Source: CAD feature listing. Evaluate the final solid. Frame: model axes, mm. Round coordinates to 2 decimals unless told otherwise and drop trailing zeros. Write each loop counter-clockwise with the first axis right and the second up, starting at its lowest first coordinate (ties: lowest second). Pieces come first, ordered by that corner, then holes. Notation, with made-up numbers: M -12.75,44.5 L 35.25,44.5 A22 ccw 35.25,69.5 Z; hole C 76,82 d3. An arc over 180 degrees is marked long. Use a Markdown table: item, result.
```python
from build123d import *

# Parameters (mm, degrees)
SKETCH_1_R      = 11.25
EXTRUDE_1_DEPTH = 15
SKETCH_2_R      = 5
EXTRUDE_2_DEPTH = 31
CHAMFER_1_SIZE  = 1
F_6_0MM_2_D     = 6


with BuildPart() as part:
    # 草图1 → 凸台-拉伸1 (new body)
    with BuildSketch(Plane(origin=(0, 0, 0), x_dir=(1, 0, 0), z_dir=(0, 1, 0))):
        with Locations(Location((0, 0, 0), (0, 0, 270))):
            Circle(SKETCH_1_R)
    extrude(amount=EXTRUDE_1_DEPTH)

    # 草图2 → 凸台-拉伸2 (add)
    with BuildSketch(Plane(origin=(0, 15, 0), x_dir=(1, 0, 0), z_dir=(0, 1, 0))):
        with Locations(Location((0, 0, 0), (0, 0, 270))):
            Circle(SKETCH_2_R)
    extrude(amount=EXTRUDE_2_DEPTH)

    # 倒角1
    chamfer_1_edges = [part.edges().sort_by_distance(p)[0] for p in [
        (0, 0, -11.25),
        (0, 15, -11.25),
    ]]
    chamfer(chamfer_1_edges, length=CHAMFER_1_SIZE)

    # Ø6.0mm 暗销孔2 (through all)
    with Locations(Plane(origin=(0, 7.5, 11.25), x_dir=(1, 0, 0), z_dir=(0, 0, 1))):
        with Locations((0, 0)):
            Hole(F_6_0MM_2_D / 2)


solid = part.part
```
Q1. Mould query, pull axis X, two halves, no side actions, for faces 1 (the cylindrical face through (-4.88, 30.28, -1.08)), 2 (the cylindrical face through (3, 7.6, -0.2)), 3 (the flat face through (5, 15, 2)). Classes: +X half, -X half, draft (parallel to the pull), parting line (faces both ways), or undercut.
Results are:
| item | result |
|---|---|
| face 1 | parting line |
| face 2 | undercut |
| face 3 | draft |
Q2. Section B-B on z = 0. Return loops of the section in (x, y).
Results are:
| item | result |
|---|---|
| outline | M -11.25,1 L -10.25,0 L 10.25,0 L 11.25,1 L 11.25,14 L 10.25,15 L 5,15 L 5,46 L -5,46 L -5,15 L -10.25,15 L -11.25,14 Z; hole C 0,7.5 d6 |
Q3. Section A-A on x = 0. Return loops of the section in (y, z), plus the area to 4 significant figures.
Results are:
| item | result |
|---|---|
| outline | M 0,-10.25 L 1,-11.25 L 4.5,-11.25 L 4.5,11.25 L 1,11.25 L 0,10.25 Z; M 10.5,-11.25 L 14,-11.25 L 15,-10.25 L 15,-5 L 46,-5 L 46,5 L 15,5 L 15,10.25 L 14,11.25 L 10.5,11.25 Z |
| area | 510.5 mm^2 |
Q4. Section C-C on y = 35. Return loops of the section in (x, z).
Results are:
| item | result |
|---|---|
| outline | C 0,0 d10 |
Q5. Section D-D on y = 7.5. Return loops of the section in (x, z).
Results are:
| item | result |
|---|---|
| outline | M -3,-10.84 L -3,10.84 A11.25 ccw Z; M 3,-10.84 A11.25 ccw 3,10.84 Z |
Q6. Line query: L1, parallel to Y at x = 0, z = -1.25; L2, parallel to X at y = 7.5, z = 0.25; L3, parallel to Y at x = -4.5, z = 2.75. Output: solid intervals per line, ascending.
Results are:
| item | result |
|---|---|
| L1 | 0 to 4.5, 10.5 to 46 |
| L2 | -11.25 to -3, 3 to 11.25 |
| L3 | 0 to 15 |
Q7. First-contact query: pin 1 Ø4 at (y, z) = (30, 4.5) entering from +X; pin 2 Ø3 at (y, z) = (10.5, -3.5) entering from +X; pin 3 Ø5 at (x, y) = (-2.5, 20.5) entering from -Z. Flat tips, straight axial feed; report the tip coordinate or a pass-through.
Results are:
| item | result |
|---|---|
| pin 1 | x = 4.33 |
| pin 2 | x = 11.07 |
| pin 3 | z = -5 |
